Could you check a few things on this model? Use its own coordinates, in mm. Face numbers are marked on the shaded views. A direction names the side the tool comes from. Round coordinates to 2 decimals unless told otherwise and drop trailing zeros. Loops run counter-clockwise (first coordinate to the right, second up) from the corner with the lowest first, then second, coordinate; pieces in that order, holes last. Notation, with made-up numbers: (-35, 42) -> (3, 42) arc R37 ccw to (3, 78) -> close; hole circle Ø5 at (-11.5, 59.5). An arc over 180 degrees is marked (long way). One line per item, written item: value.
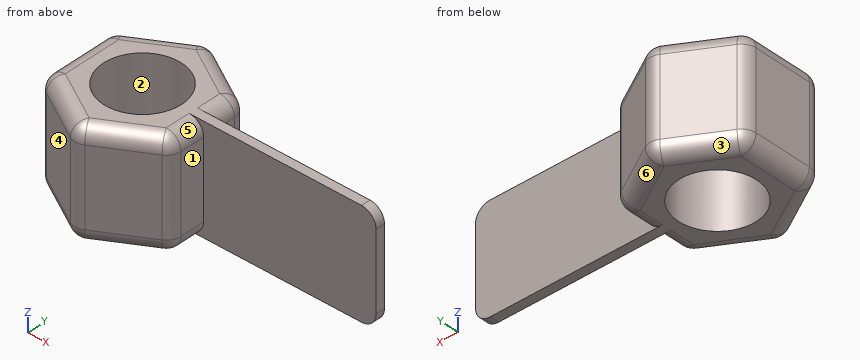
```python
from build123d import *

# Parameters (mm, degrees)
F0_R     = 13.612329
F1_DEPTH = 37.084
F2_W     = 3.215712
F2_H     = 37.084
F3_DEPTH = 60.198
F4_R     = 5.08


with BuildPart() as f1:
    # F0 (on Top) → F1 (new body)
    with BuildSketch(Plane.XY):
        Polygon((22.736654, -13.127013), (22.736654, 13.127013), (0, 26.254026), (-22.736654, 13.127013), (-22.736654, -13.127013), (0, -26.254026), align=None)
        Circle(F0_R, mode=Mode.SUBTRACT)
    extrude(amount=F1_DEPTH)

    # F2 (on face) → F3 (join)
    with BuildSketch(Plane.YZ.offset(22.736654)):
        with Locations((0.064627, 18.542)):
            Rectangle(F2_W, F2_H)
    extrude(amount=F3_DEPTH)

    # F4
    f4_edges = [f1.edges().sort_by_distance(p)[0] for p in [
        (-11.368327, -19.69052, 37.084),
        (22.736654, -7.335121, 37.084),
        (22.736654, 7.399748, 37.084),
        (11.368327, 19.69052, 37.084),
        (-11.368327, 19.69052, 37.084),
        (-22.736654, 0, 37.084),
        (11.368327, 19.69052, 0),
        (-11.368327, 19.69052, 0),
        (-22.736654, 0, 0),
        (-11.368327, -19.69052, 0),
        (11.368327, -19.69052, 0),
        (22.736654, -7.335121, 0),
        (22.736654, 7.399748, 0),
        (82.934654, 0.064627, 0),
        (82.934654, 0.064627, 37.084),
        (11.368327, -19.69052, 37.084),
        (-22.736654, 13.127013, 18.542),
        (22.736654, 13.127013, 18.542),
        (0, 26.254026, 18.542),
        (-22.736654, -13.127013, 18.542),
        (0, -26.254026, 18.542),
        (22.736654, -13.127013, 18.542),
    ]]
    fillet(f4_edges, radius=F4_R)


solid = f1.part
```
(1) For pin 1 Ø6 at (y, z) = (7.5, 28.5) entering from +X; pin 2 Ø10 at (x, z) = (9.5, 23) entering from -Y; pin 3 Ø6 at (y, z) = (16, 33) entering from +X; pin 4 Ø12 at (x, y) = (-6, 12) entering from -Z, each with a flat end and sliding along its axis, tell me the tip position at first contact or that it passes through.
Results below:
pin 1: stops at x = 22.74
pin 2: stops at y = -23.66
pin 3: stops at x = 21.83
pin 4: stops at z = 0
(2) We'd pull the mould along Y, two halves only. Please class the marked faces 1, 2, 3 and 4: +Y half, -Y half, draft (parallel to the pull), parting line (faces both ways), or undercut.
Results below:
face 1: draft
face 2: undercut
face 3: +Y half
face 4: -Y half
(3) Please list where these lines run through material, in increasing order: L1, parallel to Y at x = 0, z = 15; L2, parallel to Y at x = 28, z = 23.5; L3, parallel to X at y = -10, z = 20.5.
Results below:
L1: y = -25.47 to -13.61, 13.61 to 25.47
L2: y = -1.54 to 1.67
L3: x = -22.74 to -9.24, 9.24 to 22.74
(4) Imagine slicing it at A-A on z = 17.5. Write out the boundary of the cut face in (x, y).
Results below:
outline: (-22.74, -10.19) arc R5.08 ccw to (-20.2, -14.59) -> (-2.54, -24.79) arc R5.08 ccw to (2.54, -24.79) -> (20.2, -14.59) arc R5.08 ccw to (22.74, -10.19) -> (22.74, -1.54) -> (82.93, -1.54) -> (82.93, 1.67) -> (22.74, 1.67) -> (22.74, 10.19) arc R5.08 ccw to (20.2, 14.59) -> (2.54, 24.79) arc R5.08 ccw to (-2.54, 24.79) -> (-20.2, 14.59) arc R5.08 ccw to (-22.74, 10.19) -> close; hole circle Ø27.22 at (0, 0)
(5) Imagine slicing it at B-B on y = 0. Write out the boundary of the cut face in (x, z), then the cut area to 3 significant figures.
Results below:
outline: (-22.74, 5.08) arc R5.08 ccw to (-17.66, 0) -> (-13.61, 0) -> (-13.61, 37.08) -> (-17.66, 37.08) arc R5.08 ccw to (-22.74, 32) -> close; (13.61, 0) -> (77.85, 0) arc R5.08 ccw to (82.93, 5.08) -> (82.93, 32) arc R5.08 ccw to (77.85, 37.08) -> (13.61, 37.08) -> close
area: 2,890 mm²
(6) On a 3-axis mill with a long thin cutter (end or side, diameter ignored), from which of +Z, -Z, +X, -X, +Y, -Y can I reach the whole of each face in a straight line? I mean the marked faces 5 and 6. Say none if no direction works.
Results below:
face 5: +Z, +X, -Y
face 6: -Z, +X, +Y
(7) Imagine slicing it at C-C on x = 28. Write out the boundary of the cut face in (y, z), then the cut area to 3 significant figures.
Results below:
outline: (-1.54, 0) -> (1.67, 0) -> (1.67, 37.08) -> (-1.54, 37.08) -> close
area: 119 mm²
